```python
from build123d import *

# Parameters (mm, degrees)
SKETCH1_R               = 1.0922
SKETCH1_R_2             = 0.7922
EXTRUDE_THIN1_DEPTH     = 6.5
SKETCH5_R               = 0.7422
CUT_EXTRUDE1_DEPTH      = 2.0922
CUT_EXTRUDE1_DEPTH_BACK = 2.0922
SKETCH10_R              = 0.254
CUT_EXTRUDE5_DEPTH      = 10
CUT_EXTRUDE5_DEPTH_BACK = 10
SKETCH9_R               = 0.25
CUT_EXTRUDE4_DEPTH      = 10
CUT_EXTRUDE4_DEPTH_BACK = 10


with BuildPart() as part:
    # Sketch1 → Extrude-Thin1 (new body)
    with BuildSketch(Plane(origin=(0, 0, 0), x_dir=(1, 0, 0), z_dir=(0, 1, 0))):
        Circle(SKETCH1_R)
        Circle(SKETCH1_R_2, mode=Mode.SUBTRACT)
    extrude(amount=EXTRUDE_THIN1_DEPTH)

    # Sweep2: sweep along a path in Sketch4_2
    with BuildLine(Plane.XY) as sweep2_path:
        ThreePointArc((-1.0922, 6.5), (-1.734234713, 8.899597356), (-3.24479024, 10.87152485))
    # Sketch12 → Sweep2 (sweep)
    with BuildSketch(Plane(origin=(0, 6.5, 0), x_dir=(1, 0, 0), z_dir=(0, 1, 0))):
        with BuildLine():
            Line((-0.396875, -1.017541682), (-0.396875, -0.685617294))
            ThreePointArc((-0.396875, -0.685617294), (-0.7922, 0), (-0.396875, 0.685617294))
            Line((-0.396875, 0.685617294), (-0.396875, 1.017541682))
            ThreePointArc((-0.396875, 1.017541682), (-1.0922, 0), (-0.396875, -1.017541682))
        make_face()
    sweep2 = sweep(path=sweep2_path.line)

    # Cut-Sweep1: sweep along a path in Sketch13
    with BuildLine(Plane.XY) as cut_sweep1_path:
        ThreePointArc((-1.0922, 6.5), (-1.531167448, 8.442831006), (-2.54839741, 10.155293544))
    # Sketch14 → Cut-Sweep1 (sweep, cut)
    with BuildSketch(Plane(origin=(0, 6.5, 0), x_dir=(1, 0, 0), z_dir=(0, 1, 0))):
        with BuildLine():
            Line((-0.396875, -1.017541682), (-0.396875, -0.685617294))
            ThreePointArc((-0.396875, -0.685617294), (-0.605077108, -0.511334072), (-0.7422, -0.276983754))
            Line((-0.7422, -0.276983754), (-0.7422, -0.801273986))
            ThreePointArc((-0.7422, -0.801273986), (-0.579711905, -0.925653794), (-0.396875, -1.017541682))
        make_face()
        with BuildLine():
            Line((-0.396875, 0.685617294), (-0.396875, 1.017541682))
            ThreePointArc((-0.396875, 1.017541682), (-0.579711905, 0.925653794), (-0.7422, 0.801273986))
            Line((-0.7422, 0.801273986), (-0.7422, 0.276983754))
            ThreePointArc((-0.7422, 0.276983754), (-0.605077108, 0.511334072), (-0.396875, 0.685617294))
        make_face()
    cut_sweep1 = sweep(path=cut_sweep1_path.line, mode=Mode.SUBTRACT)

    # Mirror1: Sweep2, Cut-Sweep1 across plane
    add(sweep2.mirror(Plane(origin=(0, 0, 0), x_dir=(0, 0, 1), z_dir=(1, 0, 0))))
    add(cut_sweep1.mirror(Plane(origin=(0, 0, 0), x_dir=(0, 0, 1), z_dir=(1, 0, 0))), mode=Mode.SUBTRACT)

    # Sketch5 → Cut-Extrude1 (cut, two sides)
    with BuildSketch(Plane.XY) as cut_extrude1_sk:
        with Locations((0, 6.5)):
            Circle(SKETCH5_R)
    extrude(amount=CUT_EXTRUDE1_DEPTH, mode=Mode.SUBTRACT)
    extrude(cut_extrude1_sk.sketch, amount=-CUT_EXTRUDE1_DEPTH_BACK, mode=Mode.SUBTRACT)

    # Sketch10 → Cut-Extrude5 (cut, two sides)
    with BuildSketch(Plane.XY) as cut_extrude5_sk:
        with Locations((0.001350263, 4.3)):
            Circle(SKETCH10_R)
        with Locations((0.001426468, 3.200000003)):
            Circle(SKETCH10_R)
        with BuildLine():
            Line((0.398301468, 0.5), (0.398301468, 0))
            Line((0.398301468, 0), (-0.395448532, 0))
            Line((-0.395448532, 0), (-0.395448532, 0.5))
            ThreePointArc((-0.395448532, 0.5), (0.001426468, 0.896875), (0.398301468, 0.5))
        make_face()
    extrude(amount=CUT_EXTRUDE5_DEPTH, mode=Mode.SUBTRACT)
    extrude(cut_extrude5_sk.sketch, amount=-CUT_EXTRUDE5_DEPTH_BACK, mode=Mode.SUBTRACT)

    # Sketch9 → Cut-Extrude4 (cut, two sides)
    with BuildSketch(Plane(origin=(0, 0, 0), x_dir=(0, 0, -1), z_dir=(1, 0, 0))) as cut_extrude4_sk:
        with Locations((0, 1.5)):
            Circle(SKETCH9_R)
    extrude(amount=CUT_EXTRUDE4_DEPTH, mode=Mode.SUBTRACT)
    extrude(cut_extrude4_sk.sketch, amount=-CUT_EXTRUDE4_DEPTH_BACK, mode=Mode.SUBTRACT)


solid = part.part
```
Model file for the job. Use its own axes, mm. Round coordinates to 2 decimals unless told otherwise and drop trailing zeros. Order: outer loops, then holes, each group sorted by start corner. A loop starts at its lowest first (then second) coordinate and runs counter-clockwise, first axis right, second up. Notation, with made-up numbers: (5.5, -38) -> (14.5, -38) arc R11 cw to (14.5, -31) -> close; hole circle Ø5 at (86.5, 48.5). An arc over 180 degrees is marked (long way). Use one line per item in the form item = value.
Item 1: Cut at C-C, the plane z = 0. Give the number of separate pieces and of enclosed holes in the cut face, and give its area (3 significant figures).
Returned:
separate_pieces = 4
enclosed_holes = 0
area = 6.66 mm^2
Item 2: Cut at B-B, the plane y = 4.3. Write the cut outline in (x, z).
Returned:
outline = (-0.25, -1.06) -> (-0.25, -0.75) arc R0.79 cw to (-0.25, 0.75) -> (-0.25, 1.06) arc R1.09 ccw to start; (0.26, -1.06) arc R1.09 ccw to (0.26, 1.06) -> (0.26, 0.75) arc R0.79 cw to (0.26, -0.75) -> close
Item 3: Cut at A-A, the plane x = 0. Write the cut outline in (y, z).
Returned:
outline = (0.9, -1.09) -> (2.95, -1.09) -> (2.95, -0.79) -> (0.9, -0.79) -> close; (0.9, 0.79) -> (2.95, 0.79) -> (2.95, 1.09) -> (0.9, 1.09) -> close; (3.45, -1.09) -> (4.05, -1.09) -> (4.05, -0.79) -> (3.45, -0.79) -> close; (3.45, 0.79) -> (4.05, 0.79) -> (4.05, 1.09) -> (3.45, 1.09) -> close; (4.55, -1.09) -> (5.76, -1.09) -> (5.76, -0.79) -> (4.55, -0.79) -> close; (4.55, 0.79) -> (5.76, 0.79) -> (5.76, 1.09) -> (4.55, 1.09) -> close
Item 4: Pull direction X, two halves, no side cores. Call faces 1 (the face through (-1.187, 8.523, 0.543)), 2 (the face through (1.04, 3.2, -0.33)): released by +X, released by -X, zero draft, split by the parting line, or undercut.
Returned:
face_1 = undercut
face_2 = split by the parting line
Item 5: Cut at D-D, the plane y = 1.5. Write the cut outline in (x, z), and give its area (3 significant figures).
Returned:
outline = (-1.06, -0.25) arc R1.09 ccw to (1.06, -0.25) -> (0.75, -0.25) arc R0.79 cw to (-0.75, -0.25) -> close; (-1.06, 0.25) -> (-0.75, 0.25) arc R0.79 cw to (0.75, 0.25) -> (1.06, 0.25) arc R1.09 ccw to start
area = 1.47 mm^2
Item 6: Drill centre lines: line 1 (X direction, y = 4.3, z = -0.85); line 2 (X direction, y = 5.25, z = -0.2); line 3 (Z direction, x = -0.9, y = 1.5). Where is each one in solid material? Low to high.
Returned:
line_1 = -0.69 to -0.25, 0.26 to 0.69
line_2 = -1.07 to -0.77, 0.77 to 1.07
line_3 = -0.62 to -0.25, 0.25 to 0.62
Item 7: Flat gauge pin, fed straight in: pin 1 Ø3 at (x, y) = (0.5, 4) entering from +Z. Where does the tip first touch, or does it go through?
Returned:
pin_1 = 1.09
